CAD build for the part. Positions are in the model's coordinates, mm. Coordinates: 2 decimals unless noted, no trailing zeros. Order: outer loops, then holes, each group sorted by start corner. A loop starts at its lowest first (then second) coordinate and runs counter-clockwise, first axis right, second up. Notation, with made-up numbers: (-28.75, 18) - (22.25, 18) arc R18 ccw to (22.25, 53) - close; hole circle Ø1 at (62.5, -18). An arc over 180 degrees is marked (long way). Write each question's results on one line, items separated by ' | '. Start each with the question number.
Q1. Band-saw the part on A-A, the plane y = 26. Write the cut outline in (x, z).
Q2. Band-saw the part on C-C, the plane z = 55. Write the cut outline in (x, y), then the cut area to 3 significant figures.
Q3. Pin check, flat tip, straight feed: P1, Ø2, axis at x = -3, z = 1, coming from the -Y side. Stop position of the tip, or through.
Q4. Band-saw the part on B-B, the plane x = -32. Write the cut outline in (y, z).
Q5. Wall check: probe 1 along Z at (x, y) = (24.5, 38); probe 2 along X at (y, z) = (66.5, 82). Give the ranges that are in metal, low to high.
```python
from build123d import *

# Parameters (mm, degrees)
F1_DEPTH = 2.54
F2_R     = 1.143
F3_DEPTH = 88.9


with BuildPart() as f1:
    # F0 (on Top) → F1 (new body)
    with BuildSketch(Plane.XY):
        with BuildLine():
            Line((38.1, 68.531136), (-38.1, 68.531136))
            ThreePointArc((-38.1, 68.531136), (-40.299705, 67.261136), (-40.299705, 64.721136))
            Line((-40.299705, 64.721136), (-2.199705, -1.27))
            ThreePointArc((-2.199705, -1.27), (0, -2.54), (2.199705, -1.27))
            Line((2.199705, -1.27), (40.299705, 64.721136))
            ThreePointArc((40.299705, 64.721136), (40.299705, 67.261136), (38.1, 68.531136))
        make_face()
        Polygon((38.1, 65.991136), (0, 0), (-38.1, 65.991136), align=None, mode=Mode.SUBTRACT)
    extrude(amount=F1_DEPTH)

    # F2 (on Top) → F3 (join)
    with BuildSketch(Plane.XY):
        with Locations((0, 67.261136)):
            Circle(F2_R)
    extrude(amount=F3_DEPTH)


solid = f1.part
```
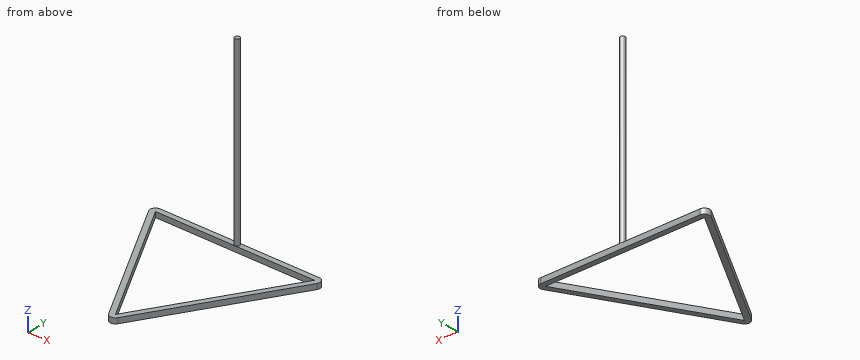
Results below:
1) outline: (-17.94, 0) - (-15.01, 0) - (-15.01, 2.54) - (-17.94, 2.54) - close; (15.01, 0) - (17.94, 0) - (17.94, 2.54) - (15.01, 2.54) - close
2) outline: circle Ø2.29 at (0, 67.26) | area: 4.10 mm²
3) P1: stops at y = -1.57
4) outline: (50.35, 0) - (55.43, 0) - (55.43, 2.54) - (50.35, 2.54) - close; (65.99, 0) - (68.53, 0) - (68.53, 2.54) - (65.99, 2.54) - close
5) probe 1: z = 0 to 2.54 | probe 2: x = -0.85 to 0.85
